Geometry check sheet. Reference: the model listing, model coordinates, mm. A direction names the side the tool comes from. Coordinates: 2 decimals unless noted, no trailing zeros. Loops run counter-clockwise (first coordinate to the right, second up) from the corner with the lowest first, then second, coordinate; pieces in that order, holes last.
from build123d import *

# Parameters (mm, degrees)
ESQUISSE1_W        = 120
ESQUISSE1_H        = 40
BOSS_EXTRU_1_DEPTH = 6
ESQUISSE2_W        = 50
ESQUISSE2_H        = 6
BOSS_EXTRU_2_DEPTH = 6


with BuildPart() as part:
    # Esquisse1 → Boss.-Extru.1 (new body)
    with BuildSketch(Plane.XY):
        Rectangle(ESQUISSE1_W, ESQUISSE1_H)
    extrude(amount=BOSS_EXTRU_1_DEPTH)

    # Esquisse2 → Boss.-Extru.2 (add)
    with BuildSketch(Plane.XY.offset(6)):
        with Locations((0, 23)):
            Rectangle(ESQUISSE2_W, ESQUISSE2_H)
        with Locations((0, -23)):
            Rectangle(ESQUISSE2_W, ESQUISSE2_H)
    extrude(amount=-BOSS_EXTRU_2_DEPTH)


solid = part.part
(1) Access from +Z, -Z, +X, -X, +Y, -Y to the whole of each face (thin tool, end or side, straight path). Record for faces 1 (the flat face through (25, -23, 3)), 2 (the flat face through (-25, -23, 3)), 3 (the flat face through (-25, 23, 3)), 4 (the flat face through (25, 23, 3)), 5 (the flat face through (-1, 0, 6)).
Findings:
face 1: +Z, -Z, +X, -Y
face 2: +Z, -Z, -X, -Y
face 3: +Z, -Z, -X, +Y
face 4: +Z, -Z, +X, +Y
face 5: +Z, +X, -X, +Y, -Y
(2) Sectioned sample at C-C on y = -23. Record the cut outline in (x, z).
Findings:
outline: (-25, 0) - (25, 0) - (25, 6) - (-25, 6) - close
(3) Sectioned sample at A-A on z = 1.05. Record the cut outline in (x, y).
Findings:
outline: (-60, -20) - (-25, -20) - (-25, -26) - (25, -26) - (25, -20) - (60, -20) - (60, 20) - (25, 20) - (25, 26) - (-25, 26) - (-25, 20) - (-60, 20) - close
(4) Scan lines: L1, parallel to Y at x = -27.5, z = 5.45; L2, parallel to X at y = 23.5, z = 3.95. Record each from-to range of solid material in increasing order.
Findings:
L1: y = -20 to 20
L2: x = -25 to 25
(5) Sectioned sample at B-B on x = -41. Record the cut outline in (y, z), and give its area (3 significant figures).
Findings:
outline: (-20, 0) - (20, 0) - (20, 6) - (-20, 6) - close
area: 240 mm2
(6) Gauge pin test, flat ends, axial feed: pin 1 Ø3 at (y, z) = (-24, 2) entering from +X; pin 2 Ø4 at (x, y) = (25.5, -12) entering from -Z; pin 3 Ø3 at (y, z) = (24, 2) entering from -X; pin 4 Ø3 at (x, z) = (-49, 2.5) entering from -Y. Record the tip position at first contact, or that the pin passes through.
Findings:
pin 1: stops at x = 25
pin 2: stops at z = 0
pin 3: stops at x = -25
pin 4: stops at y = -20
